CAD build for the part. Positions are in the model's coordinates, mm. Face numbers are marked on the shaded views. A direction names the side the tool comes from. Round coordinates to 2 decimals unless told otherwise and drop trailing zeros. Loops run counter-clockwise (first coordinate to the right, second up) from the corner with the lowest first, then second, coordinate; pieces in that order, holes last.
Autodesk Inventor part; units mm, degrees
ref_plane "YZ Plane" through (0, 0, 0) normal (1, 0, 0) x (0, 1, 0)
ref_plane "XZ Plane" through (0, 0, 0) normal (0, 1, 0) x (-1, 0, 0)
ref_plane "XY Plane" through (0, 0, 0) normal (0, 0, 1) x (1, 0, 0)
sketch "Sketch1" plane through (0, 0, 0) normal (0, 1, 0) x (-1, 0, 0)
  circle A0 centre (0, 0) radius 335
  line L0 (335, 0) -> (-335, 0)
  line L1 (0, -335) -> (0, 335)
  line L2 (0, 0) -> (-236.8808, 236.8808)
  line L3 (0, 0) -> (236.8808, -236.8808)
  line L4 (0, 0) -> (236.8808, 236.8808)
  line L5 (0, 0) -> (-236.8808, -236.8808)
  circle A1 centre (0, 0) radius 135
  point P0 (-95.4594, 95.4594)
  point P1 (0, 135)
  dimension "d0" = 670
  dimension "d1" = 45
  dimension "d2" = 45
  dimension "d17" = 200
extrude "Extrusion1" add sketch "Sketch1" along normal blind 70 contours L1 A1 L2 A0
sketch "Sketch2" plane through (95.4594, 0, 95.4594) normal (0.7071068, 0, -0.7071068) x (-0.7071068, 0, -0.7071068)
  line L0 (-190, 60) -> (-10, 60)
  line L1 (-10, 60) -> (-10, 10)
  line L2 (-10, 10) -> (-190, 10)
  line L3 (-190, 10) -> (-190, 60)
  line L4 (-200, 0) -> (0, 0)
  line L5 (-200, 70) -> (0, 70)
  line L6 (-200, 0) -> (-200, 70)
  line L7 (0, 0) -> (0, 70)
  point P0 (135, 0)
  point P1 (0, 35)
  dimension "d6" = 10
  dimension "d7" = 10
  dimension "d8" = 10
  dimension "d9" = 10
sketch3d "3D Sketch1"
  arc A0 (95.4594, 70, 95.4594) -> (0, 70, 135) centre (0, 70, 0) ccw
sweep "Sweep1" cut profiles "Sketch2" path "3D Sketch1" contours L0 L1 L2 L3
sketch "Sketch3" plane through (95.4594, 0, 95.4594) normal (0.7071068, 0, -0.7071068) x (-0.7071068, 0, -0.7071068)
  line L0 (-101.8808, 70) -> (-200, 70)
  line L1 (32.4695, 60) -> (-94.8097, 60)
  line L2 (-145, 70) -> (-45, 70)
  line L3 (-45, 70) -> (-45, 60)
  line L4 (-45, 60) -> (-145, 60)
  line L5 (-145, 60) -> (-145, 70)
  line L6 (-200, 0) -> (-200, 70)
  line L7 (0, 0) -> (0, 70)
  point P0 (135, 0)
  dimension "d16" = 100
  dimension "d18" = 45
sketch3d "3D Sketch2"
  arc A0 (95.4594, 70, 95.4594) -> (0, 70, 135) centre (0, 70, 0) ccw
sweep "Sweep2" cut profiles "Sketch3" path "3D Sketch2"
properties part number "Carousel Fixed Track"
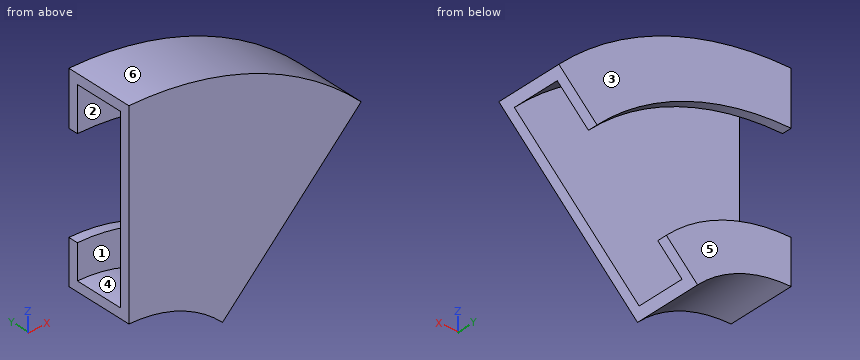
Item 1: Flat gauge pins, fed straight in: P1, Ø10, axis at x = 30, y = 47, coming from the +Z side; P2, Ø2, axis at x = 198.5, y = 48, coming from the -Z side; P3, Ø3, axis at x = 176, y = 60.5, coming from the -Z side. Where does each tip first touch, or does it go through?
Answers follow:
P1: stops at z = 334.07
P2: stops at z = 256.56
P3: stops at z = 216.55
Item 2: Probe line 1 (Y direction, x = 226, z = 231); line 2 (Y direction, x = 35, z = 277); line 3 (Z direction, x = 34.5, y = 12). List the from-to ranges inside material, lowest first.
Answers follow:
line 1: y = 0 to 10, 60 to 70
line 2: y = 0 to 10
line 3: z = 130.52 to 140.84, 323.16 to 333.22
Item 3: Cut at D-D, the plane x = 36. Give the cut face in (y, z).
Answers follow:
outline: (0, 130.11) - (70, 130.11) - (70, 176.36) - (60, 176.36) - (60, 140.46) - (10, 140.46) - (10, 323) - (60, 323) - (60, 277.68) - (70, 277.68) - (70, 333.06) - (0, 333.06) - close
Item 4: Cut at C-C, the plane y = 48. Give the cut face in (x, z), plus the area to 3 significant figures.
Answers follow:
outline: (0, 135) arc R135 cw to (95.46, 95.46) - (102.53, 102.53) arc R145 ccw to (0, 145) - close; (0, 325) arc R325 cw to (229.81, 229.81) - (236.88, 236.88) arc R335 ccw to (0, 335) - close
area: 3,690 mm2
Item 5: Cut at B-B, the plane x = 116. Give the cut face in (y, z).
Answers follow:
outline: (0, 116) - (10, 116) - (10, 303.59) - (60, 303.59) - (60, 254.84) - (70, 254.84) - (70, 314.28) - (0, 314.28) - close; (60, 116) - (70, 116) - (70, 137.64) - (60, 137.64) - close
Item 6: Cut at A-A, the plane z = 205. Give the cut face in (x, y).
Answers follow:
outline: (0, 0) - (205, 0) - (205, 10) - (0, 10) - close; (190.72, 60) - (205, 60) - (205, 70) - (190.72, 70) - close
Item 7: Two-plate mould, pull along Y, no slides. Class the marked faces 4, 5 and 6: released by +Y, released by -Y, zero draft, split by the parting line, or undercut.
Answers follow:
face 4: undercut
face 5: released by +Y
face 6: zero draft
Item 8: 3-axis set-ups, long thin cutter, end or side, ignore diameter. For the marked faces 1, 2 and 3: which of +Z, -Z, +X, -X, +Y, -Y reach the whole face in a straight line?
Answers follow:
face 1: +X
face 2: -X
face 3: +Z, -Z, +X, -X, +Y
